```python
from build123d import *

# Parameters (mm, degrees)
BASE_FLANGE1_DEPTH           = 2.65684
SKETCHED_BEND3_DEPTH         = 355.6
SKETCHED_BEND3_2_DEPTH       = 355.6
SKETCH10_R                   = 6.35
CUT_EXTRUDE2_DEPTH           = 2.65684
EDGE_FLANGE5_DEPTH           = 254
EDGE_FLANGE6_STRIP_W         = 16.97736
EDGE_FLANGE6_STRIP_H         = 2.65684
EDGE_FLANGE6_STRIP_CUT_DEPTH = 116.5225
EDGE_FLANGE6_DEPTH           = 116.5225
EDGE_FLANGE7_DEPTH           = 248.16816
SKETCH34_R                   = 6.35
CUT_EXTRUDE3_DEPTH           = 2.65684
SKETCH38_R                   = 2.032
CUT_EXTRUDE4_DEPTH           = 2.65684
SKETCH39_R                   = 2.032
CUT_EXTRUDE5_DEPTH           = 2.65684
SKETCH40_R                   = 6.35
CUT_EXTRUDE6_DEPTH           = 2.65684


# Read off the part's stored shape, not the designer's step: Sketched Bend3
# Sheet-metal steps are written as plain solids
with BuildPart() as part:
    # Sketch1 → Base-Flange1 (new body)
    with BuildSketch(Plane.XY):
        with BuildLine():
            Line((0, 0), (0, 254))
            Line((0, 254), (165.1, 254))
            ThreePointArc((165.1, 254), (177.8, 241.3), (190.5, 254))
            Line((190.5, 254), (355.6, 254))
            Line((355.6, 254), (355.6, 0))
            Line((355.6, 0), (355.6, -57.15))
            Line((355.6, -57.15), (0, -57.15))
            Line((0, -57.15), (0, 0))
        make_face()
    extrude(amount=-BASE_FLANGE1_DEPTH)

    # Sketched Bend3 outline → Sketched Bend3 (cut)
    with BuildSketch(Plane.YZ):
        with BuildLine():
            ThreePointArc((0, -2.65684), (-2.783367186, -1.949765838), (-4.891802611, 0))
            Line((-4.891802611, 0), (-57.15, 0))
            Line((-57.15, 0), (-57.15, -2.65684))
            Line((-57.15, -2.65684), (0, -2.65684))
        make_face()
    extrude(amount=SKETCHED_BEND3_DEPTH, mode=Mode.SUBTRACT)

    # Sketched Bend3 2 outline → Sketched Bend3 2 (add)
    with BuildSketch(Plane.YZ):
        with BuildLine():
            ThreePointArc((0, 0), (-2.24506403, 0.92993597), (-3.175, 3.175))
            Line((-3.175, 3.175), (-3.175, 53.251044406))
            Line((-3.175, 53.251044406), (-5.83184, 53.251044406))
            Line((-5.83184, 53.251044406), (-5.83184, 3.175))
            ThreePointArc((-5.83184, 3.175), (-5.591894488, 1.519381136), (-4.891802611, 0))
            Line((-4.891802611, 0), (0, 0))
        make_face()
    extrude(amount=SKETCHED_BEND3_2_DEPTH)

    # Sketch10 → Cut-Extrude2 (cut)
    with BuildSketch(Plane(origin=(0, -3.175, 0), x_dir=(1, 0, 0), z_dir=(0, 1, 0))):
        with Locations(Location((317.5, -34.201044406, 0), (0, 0, 270))):
            Circle(SKETCH10_R)
        with Locations(Location((247.65, -34.201044406, 0), (0, 0, 270))):
            Circle(SKETCH10_R)
        with Locations(Location((38.1, -34.201044406, 0), (0, 0, 270))):
            Circle(SKETCH10_R)
        with Locations(Location((107.95, -34.201044406, 0), (0, 0, 270))):
            Circle(SKETCH10_R)
        with Locations(Location((177.8, -34.201044406, 0), (0, 0, 270))):
            Circle(SKETCH10_R)
    extrude(amount=-CUT_EXTRUDE2_DEPTH, mode=Mode.SUBTRACT)

    # Edge-Flange5 section (across the edge) → Edge-Flange5 (add)
    with BuildSketch(Plane(origin=(-3.175, 0, -2.65684), x_dir=(1, 0, 0), z_dir=(0, 1, 0))):
        with BuildLine():
            Line((-2.65684, 3.175), (-2.65684, 119.6975))
            Line((-2.65684, 119.6975), (0, 119.6975))
            Line((0, 119.6975), (0, 3.175))
            ThreePointArc((0, 3.175), (0.92993597, 0.92993597), (3.175, 0))
            Line((3.175, 0), (3.175, -2.65684))
            ThreePointArc((3.175, -2.65684), (-0.948733611, -0.948733611), (-2.65684, 3.175))
        make_face()
    extrude(amount=EDGE_FLANGE5_DEPTH)

    # Edge-Flange6 strip (across the edge) → Edge-Flange6 strip cut (cut)
    with BuildSketch(Plane(origin=(-5.83184, 254, -5.83184), x_dir=(0, -1, 0), z_dir=(0, 0, -1))):
        with Locations((-2.65684, -1.32842)):
            Rectangle(EDGE_FLANGE6_STRIP_W, EDGE_FLANGE6_STRIP_H)
    extrude(amount=EDGE_FLANGE6_STRIP_CUT_DEPTH, mode=Mode.SUBTRACT)

    # Edge-Flange6 section (across the edge) → Edge-Flange6 (add)
    with BuildSketch(Plane(origin=(-5.83184, 254, -5.83184), x_dir=(0, -1, 0), z_dir=(0, 0, -1))):
        with BuildLine():
            Line((0, 3.175), (0, 53.975))
            Line((0, 53.975), (2.65684, 53.975))
            Line((2.65684, 53.975), (2.65684, 3.175))
            ThreePointArc((2.65684, 3.175), (3.58677597, 0.92993597), (5.83184, 0))
            Line((5.83184, 0), (5.83184, -2.65684))
            ThreePointArc((5.83184, -2.65684), (1.708106389, -0.948733611), (0, 3.175))
        make_face()
    extrude(amount=EDGE_FLANGE6_DEPTH)

    # Edge-Flange7 section (across the edge) → Edge-Flange7 (add)
    with BuildSketch(Plane(origin=(-3.175, 0, -125.52934), x_dir=(0, 0, 1), z_dir=(0, 1, 0))):
        with BuildLine():
            Line((-2.65684, 3.175), (-2.65684, 25.4))
            Line((-2.65684, 25.4), (0, 25.4))
            Line((0, 25.4), (0, 3.175))
            ThreePointArc((0, 3.175), (0.92993597, 0.92993597), (3.175, 0))
            Line((3.175, 0), (3.175, -2.65684))
            ThreePointArc((3.175, -2.65684), (-0.948733611, -0.948733611), (-2.65684, 3.175))
        make_face()
    extrude(amount=EDGE_FLANGE7_DEPTH)

    # Sketch34 → Cut-Extrude3 (cut)
    with BuildSketch(Plane(origin=(0, 254, 0), x_dir=(1, 0, 0), z_dir=(0, 1, 0))):
        with Locations(Location((-40.75684, 90.60434, 0), (0, 0, 180))):
            Circle(SKETCH34_R)
        with Locations(Location((-40.75684, 34.40684, 0), (0, 0, 180))):
            Circle(SKETCH34_R)
    extrude(amount=-CUT_EXTRUDE3_DEPTH, mode=Mode.SUBTRACT)

    # Sketch38 → Cut-Extrude4 (cut)
    with BuildSketch(Plane(origin=(0, 0, -128.18618), x_dir=(-1, 0, 0), z_dir=(0, 0, -1))):
        with Locations((-15.875, 239.27816)):
            Circle(SKETCH38_R)
        with Locations((-15.875, 213.87816)):
            Circle(SKETCH38_R)
        with Locations((-15.875, 188.47816)):
            Circle(SKETCH38_R)
        with Locations((-15.875, 163.07816)):
            Circle(SKETCH38_R)
        with Locations((-15.875, 137.67816)):
            Circle(SKETCH38_R)
        with Locations((-15.875, 112.27816)):
            Circle(SKETCH38_R)
        with Locations((-15.875, 86.87816)):
            Circle(SKETCH38_R)
        with Locations((-15.875, 61.47816)):
            Circle(SKETCH38_R)
        with Locations((-15.875, 36.07816)):
            Circle(SKETCH38_R)
        with Locations((-15.875, 10.67816)):
            Circle(SKETCH38_R)
    extrude(amount=-CUT_EXTRUDE4_DEPTH, mode=Mode.SUBTRACT)

    # Sketch39 → Cut-Extrude5 (cut)
    with BuildSketch(Plane.XY):
        with Locations((339.725, 10.67816)):
            Circle(SKETCH39_R)
        with Locations((339.725, 36.07816)):
            Circle(SKETCH39_R)
        with Locations((339.725, 61.47816)):
            Circle(SKETCH39_R)
        with Locations((339.725, 86.87816)):
            Circle(SKETCH39_R)
        with Locations((339.725, 112.27816)):
            Circle(SKETCH39_R)
        with Locations((339.725, 137.67816)):
            Circle(SKETCH39_R)
        with Locations((339.725, 163.07816)):
            Circle(SKETCH39_R)
        with Locations((339.725, 188.47816)):
            Circle(SKETCH39_R)
        with Locations((339.725, 213.87816)):
            Circle(SKETCH39_R)
        with Locations((339.725, 239.27816)):
            Circle(SKETCH39_R)
    extrude(amount=-CUT_EXTRUDE5_DEPTH, mode=Mode.SUBTRACT)

    # Sketch40 → Cut-Extrude6 (cut)
    with BuildSketch(Plane.ZY.offset(5.83184)):
        with Locations((-34.40684, 41.79316)):
            Circle(SKETCH40_R)
        with Locations((-90.28684, 41.79316)):
            Circle(SKETCH40_R)
    extrude(amount=-CUT_EXTRUDE6_DEPTH, mode=Mode.SUBTRACT)


solid = part.part
```
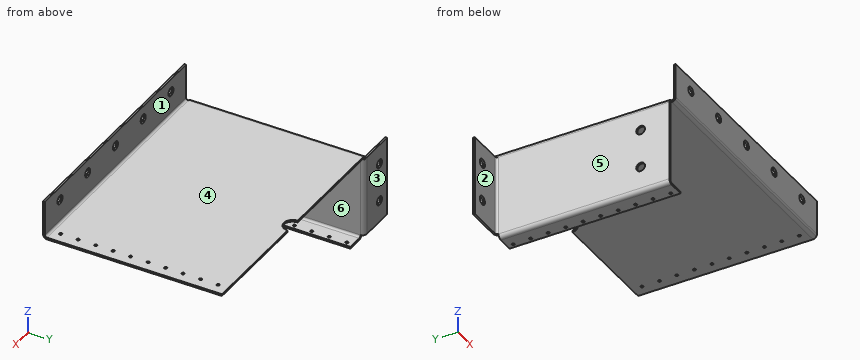
Can you work these out from the model? Positions are in its coordinate system, mm. Face numbers are marked on the shaded views. A direction names the side the tool comes from. Round coordinates to 2 decimals unless told otherwise and drop trailing zeros. Loops run counter-clockwise (first coordinate to the right, second up) from the corner with the lowest first, then second, coordinate; pieces in that order, holes last. Notation, with made-up numbers: (-18.75, 73) -> (19.25, 73) arc R24 ccw to (19.25, 106) -> close; hole circle Ø6 at (45, 37). An arc over 180 degrees is marked (long way). One line per item, written item: value. Start each with the question number.
1. If we section it at B-B, the plane y = 156: Write out the boundary of the cut face in (x, z) (3 decimals).
2. If we section it at A-A, the plane x = 107.95: Write out the boundary of the cut face in (y, z) (3 decimals).
3. If we section it at C-C, the plane x = 299: Write out the boundary of the cut face in (y, z) (3 decimals).
4. If we section it at D-D, the plane z = 35.5: Write out the boundary of the cut face in (x, y) (3 decimals).
5. If I drill on probe 1 along Z at (x, y) = (12.5, 143.5); probe 2 along Y at (x, z) = (-14.5, -101); probe 3 along Z at (x, y) = (253, 210), over which ranges is the centre line in solid material (lowest first)?
6. If we mould it in two halves opening along Z, with no side actions, what happens to the marked faces 4, 5 and 6? For each: pulls with the +Z half, pulls with the -Z half, needs draft (parallel to the pull), parting line crosses it, or undercut.
7. For pin 1 (14.5 mm diameter, centred on x = 177.8, z = 34.2, fed in from -Y); pin 2 (1 mm diameter, centred on x = 102.5, y = 76.5, fed in from -Z); pin 3 (14.5 mm diameter, centred on x = 247.65, z = 34.2, fed in from +Y) (3 decimals); pin 4 (3 mm diameter, centred on y = -4, z = 37, fed in from -X), each with a flat end and sliding along its axis, tell me the tip position at first contact or that it passes through.
8. For the marked faces 1, 2 and 3, which set-ups out of +Z, -Z, +X, -X, +Y, -Y let a thin tool reach every point of the face, with its end or its side?
Calculated:
1. outline: (-5.832, -122.354) arc R5.832 ccw to (0, -128.186) -> (22.225, -128.186) -> (22.225, -125.529) -> (0, -125.529) arc R3.175 cw to (-3.175, -122.354) -> (-3.175, -5.832) arc R3.175 cw to (0, -2.657) -> (355.6, -2.657) -> (355.6, 0) -> (0, 0) arc R5.832 ccw to (-5.832, -5.832) -> close
2. outline: (-5.832, 3.175) arc R5.832 ccw to (0, -2.657) -> (254, -2.657) -> (254, 0) -> (0, 0) arc R3.175 cw to (-3.175, 3.175) -> (-3.175, 27.851) -> (-5.832, 27.851) -> close; (-5.832, 40.551) -> (-3.175, 40.551) -> (-3.175, 53.251) -> (-5.832, 53.251) -> close
3. outline: (-5.832, 3.175) arc R5.832 ccw to (0, -2.657) -> (254, -2.657) -> (254, 0) -> (0, 0) arc R3.175 cw to (-3.175, 3.175) -> (-3.175, 53.251) -> (-5.832, 53.251) -> close
4. outline: (0, -5.832) -> (31.884, -5.832) -> (31.884, -3.175) -> (0, -3.175) -> close; (44.316, -5.832) -> (101.734, -5.832) -> (101.734, -3.175) -> (44.316, -3.175) -> close; (114.166, -5.832) -> (171.584, -5.832) -> (171.584, -3.175) -> (114.166, -3.175) -> close; (184.016, -5.832) -> (241.434, -5.832) -> (241.434, -3.175) -> (184.016, -3.175) -> close; (253.866, -5.832) -> (311.284, -5.832) -> (311.284, -3.175) -> (253.866, -3.175) -> close; (323.716, -5.832) -> (355.6, -5.832) -> (355.6, -3.175) -> (323.716, -3.175) -> close
5. probe 1: z = -128.19 to -125.53, -2.66 to 0
5. probe 2: y = 251.34 to 254
5. probe 3: z = -2.66 to 0
6. face 4: pulls with the +Z half
6. face 5: needs draft
6. face 6: undercut
7. pin 1: stops at y = -5.83
7. pin 2: stops at z = -2.66
7. pin 3: stops at y = -3.175
7. pin 4: stops at x = 0
8. face 1: +Z, +X, -X, +Y
8. face 2: +Z, -Z, -X, -Y
8. face 3: +Z, -Z, +X, -X, +Y
